The listing builds one solid part. Answer for the finished solid, in the listing's coordinates (mm). Face numbers are marked on the shaded views. A direction names the side the tool comes from. Give positions to 0.01 mm unless a question says otherwise; leave off trailing zeros. Loops run counter-clockwise (first coordinate to the right, second up) from the corner with the lowest first, then second, coordinate; pieces in that order, holes last. Notation, with made-up numbers: M -36.5,-26 L -29.5,-26 A14 cw -29.5,-17 Z; hole C 60,-24.75 d11. An arc over 180 degrees is marked long. Use one line per item in the form item = value. Start each with the question number.
1. For the marked faces 4 and 5, determine the directions among +Z, -Z, +X, -X, +Y, -Y from which every point of the face is accessible in a straight line to the end or side of a thin tool.
2. The part is cut by section D-D (y = 41). Write down the section's boundary in (x, z), and give its area (3 significant figures).
3. The part is cut by section A-A (y = 11.5). Give the number of separate pieces and of enclosed holes in the cut face, and give its area (3 significant figures).
4. The part is cut by section C-C (y = 24). Write down the section's boundary in (x, z).
5. Straight lines are drawn through the part: line 1 (X direction, y = 51.5, z = 9.5); line 2 (Z direction, x = 10.5, y = 25); line 3 (X direction, y = 5, z = -37.5) (3 decimals). For each, find the intervals that lie inside material, in ascending order. Write a range as from..to.
6. Each of these flat-tipped pins is pushed along its axis until it touches: pin 1 Ø1.5 at (x, z) = (-37, 26.5) entering from -Y; pin 2 Ø0.6 at (x, y) = (57, 20.5) entering from +Z; pin 3 Ø1.6 at (x, y) = (-56.5, 12.5) entering from +Z. Where does it stop, or does it pass through?
7. The mould has two halves that part along X. Classify the marked faces 1, 2 and 3: released by +X, released by -X, zero draft, split by the parting line, or undercut.
8. The part is cut by section B-B (z = -18). Write down the section's boundary in (x, y), and give its area (3 significant figures).
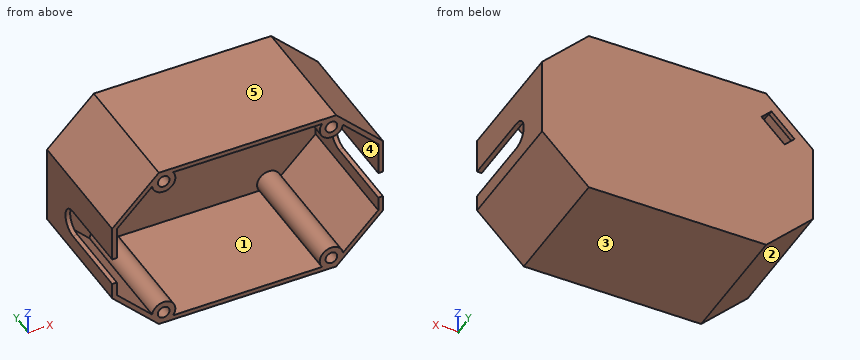
from build123d import *

# Parameters (mm, degrees)
BOSS_EXTRUDE1_DEPTH = 52
BOSS_EXTRUDE2_DEPTH = 2
SKETCH3_R           = 5
BOSS_EXTRUDE3_DEPTH = 52
SKETCH4_R           = 2.5
CUT_EXTRUDE1_DEPTH  = 15
CUT_EXTRUDE2_DEPTH  = 15
CUT_EXTRUDE3_REACH  = 136.539


with BuildPart() as part:
    # Sketch1 → Boss-Extrude1 (new body)
    with BuildSketch(Plane(origin=(0, 0, 0), x_dir=(1, 0, 0), z_dir=(0, 1, 0))):
        Polygon((38, -32.421617333), (-38, -32.421617333), (-58, -12.421649809), (-58, 21.578350191), (-38, 41.578382667), (38, 41.578382667), (58, 21.578415143), (58, -12.421584857), align=None)
        Polygon((-37.171571924, 39.578382667), (-56, 20.749924017), (-56, -11.593221733), (-37.171573826, -30.421617333), (37.171571924, -30.421617333), (56, -11.593158683), (56, 20.749987067), (37.171573826, 39.578382667), align=None, mode=Mode.SUBTRACT)
    extrude(amount=BOSS_EXTRUDE1_DEPTH)

    # Sketch2 → Boss-Extrude2 (add)
    with BuildSketch(Plane(origin=(0, 52, 0), x_dir=(1, 0, 0), z_dir=(0, 1, 0))):
        Polygon((38, -32.421617333), (58, -12.421584857), (58, 21.578415143), (38, 41.578382667), (-38, 41.578382667), (-58, 21.578350191), (-58, -12.421649809), (-38, -32.421617333), align=None)
    extrude(amount=BOSS_EXTRUDE2_DEPTH)

    # Sketch3 → Boss-Extrude3 (add)
    with BuildSketch(Plane.XZ.offset(-52)):
        with Locations((35.928934566, -36.578382667)):
            Circle(SKETCH3_R)
        with Locations((-35.92892981, -36.578382667)):
            Circle(SKETCH3_R)
        with Locations((-35.928934566, 27.421617333)):
            Circle(SKETCH3_R)
        with Locations((35.92892981, 27.421617333)):
            Circle(SKETCH3_R)
    extrude(amount=BOSS_EXTRUDE3_DEPTH)

    # Sketch4 → Cut-Extrude1 (cut)
    with BuildSketch(Plane(origin=(0, 0, 0), x_dir=(-1, 0, 0), z_dir=(0, -1, 0))):
        with Locations(Location((-35.928934566, 36.578382667, 0), (0, 0, 90))):
            Circle(SKETCH4_R)
        with Locations(Location((35.92892981, 36.578382667, 0), (0, 0, 90))):
            Circle(SKETCH4_R)
        with Locations(Location((35.928934566, -27.421617333, 0), (0, 0, 90))):
            Circle(SKETCH4_R)
        with Locations(Location((-35.92892981, -27.421617333, 0), (0, 0, 90))):
            Circle(SKETCH4_R)
    extrude(amount=-CUT_EXTRUDE1_DEPTH, mode=Mode.SUBTRACT)

    # Sketch5 → Cut-Extrude2 (cut)
    with BuildSketch(Plane(origin=(0, 54, 0), x_dir=(1, 0, 0), z_dir=(0, 1, 0))):
        Polygon((-50.121326659, -14.6434607), (-40.221823685, -24.5429476), (-35.979186442, -20.300303468), (-45.878689416, -10.400816569), align=None)
    extrude(amount=-CUT_EXTRUDE2_DEPTH, mode=Mode.SUBTRACT)

    # Cut-Extrude3: up to this face of the body (flat: up to its plane)
    cut_extrude3_end = Plane(part.part.faces().sort_by_distance((58, 27, -4.578415143))[0])
    # Sketch6 → Cut-Extrude3 (cut, up to the picked face)
    with BuildSketch(Plane.ZY.offset(58), mode=Mode.PRIVATE) as cut_extrude3_sk1:
        with BuildLine():
            Line((-14.578350191, 0), (-14.578350191, 32.713069052))
            ThreePointArc((-14.578350191, 32.713069052), (-8.578350191, 38.713069052), (-2.578350191, 32.713069052))
            Line((-2.578350191, 32.713069052), (-2.578350191, 0))
            Line((-2.578350191, 0), (-14.578350191, 0))
        make_face()
    cut_extrude3_tool1 = split(extrude(cut_extrude3_sk1.sketch, amount=-CUT_EXTRUDE3_REACH, mode=Mode.PRIVATE), bisect_by=cut_extrude3_end, keep=Keep.BOTH, mode=Mode.PRIVATE)
    add(cut_extrude3_tool1.solids().sort_by(Axis((-58, 18.736689, -8.57835), (1, 0, 0)))[0], mode=Mode.SUBTRACT)


solid = part.part
Derived:
q1.face_4 = -Y
q1.face_5 = +Z, +X, -X, +Y, -Y
q2.outline = M -58,-21.58 L -38,-41.58 L 38,-41.58 L 58,-21.58 L 58,12.42 L 38,32.42 L -38,32.42 L -58,12.42 Z; hole M -56,-20.75 L -40.88,-35.87 A5 cw long -31.93,-39.58 L 31.93,-39.58 A5 cw long 40.88,-35.87 L 56,-20.75 L 56,11.59 L 40.88,26.71 A5 cw long 31.93,30.42 L -31.93,30.42 A5 cw long -40.88,26.71 L -56,11.59 Z
q2.area = 898 mm2
q3.separate_pieces = 2
q3.enclosed_holes = 4
q3.area = 772 mm2
q4.outline = M -58,-21.58 L -38,-41.58 L 38,-41.58 L 58,-21.58 L 58,-14.58 L 56,-14.58 L 56,-20.75 L 40.88,-35.87 A5 ccw long 31.93,-39.58 L -31.93,-39.58 A5 ccw long -40.88,-35.87 L -56,-20.75 L -56,-14.58 L -58,-14.58 Z; M -58,-2.58 L -56,-2.58 L -56,11.59 L -40.88,26.71 A5 ccw long -31.93,30.42 L 31.93,30.42 A5 ccw long 40.88,26.71 L 56,11.59 L 56,-2.58 L 58,-2.58 L 58,12.42 L 38,32.42 L -38,32.42 L -58,12.42 Z
q5.line_1 = -58..-56, 56..58
q5.line_2 = -41.58..-39.58, 30.42..32.42
q5.line_3 = -42.078..-38.253, -33.605..-31.015, 31.015..33.605, 38.253..42.078
q6.pin_1 = 15
q6.pin_2 = 13.72
q6.pin_3 = 14.72
q7.face_1 = undercut
q7.face_2 = released by -X
q7.face_3 = zero draft
q8.outline = M -58,0 L -56,0 L -56,52 L 56,52 L 56,0 L 58,0 L 58,54 L -58,54 Z
q8.area = 440 mm2
